Study the drawing (mm; zero at the part's minimum x, y, z) and answer. Round coordinates to 2 decimals unless told otherwise and drop trailing zeros. Loops run counter-clockwise (first coordinate to the right, second up) from the corner with the lowest first, then second, coordinate; pieces in that order, holes last. Notation, with made-up numbers: (85, -1.75) -> (102, -1.75) arc R27 cw to (102, 20.25) -> close; hole circle Ø1 at (84.25, 6.25). An arc over 180 degrees is marked (long way). Answer in a Markdown table with one row per item. Add a question column.
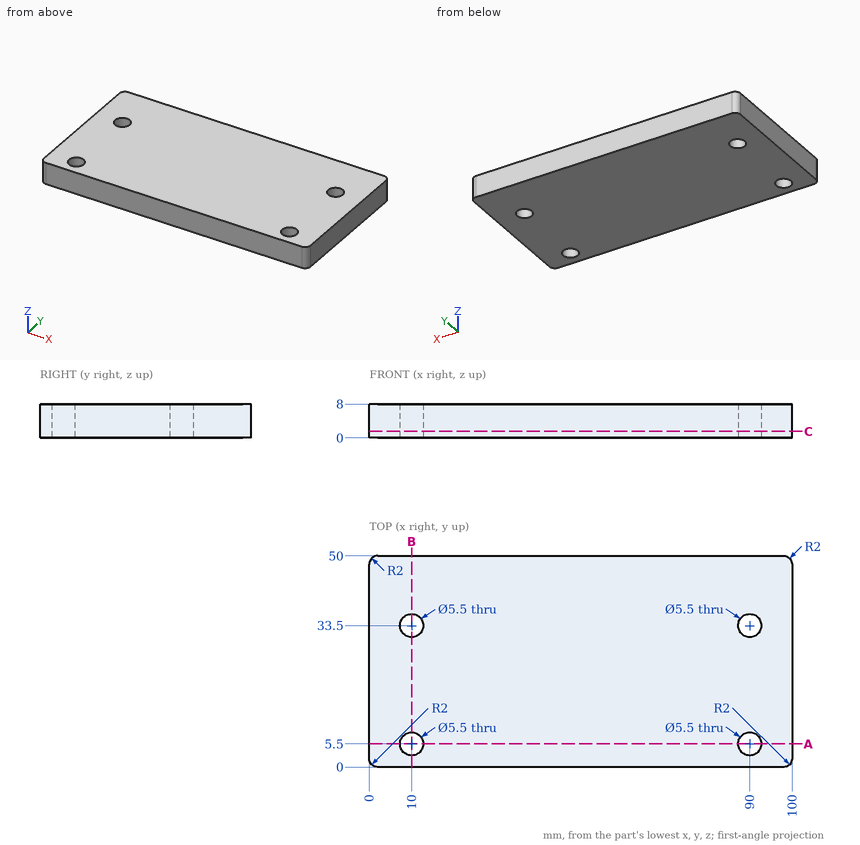
Item 1: Section A-A, the plane y = 5.5 is taken. Write down the section's boundary in (x, z).
Item 2: A flat-ended cylindrical pin translates along its axis: P1, Ø5, axis at x = 10, y = 33.5, coming from the -Z side. Find the tip coordinate at first contact, or state that the pin passes through.
Item 3: Section B-B, the plane x = 10 is taken. Write down the section's boundary in (y, z), and give its area (3 significant figures).
Item 4: Section C-C, the plane z = 1.5 is taken. Write down the section's boundary in (x, y), and give its area (3 significant figures).
Item 5: Consider L1, parallel to X at y = 33.5, z = 5; L2, parallel to Y at x = 90, z = 6; L3, parallel to X at y = 3, z = 0.5. Determine where each line is inside the solid, lowest interval first. Write a range as from..to.
Here are the results:
| question | item | result |
|---|---|---|
| 1 | outline | (0, 0) -> (7.25, 0) -> (7.25, 8) -> (0, 8) -> close; (12.75, 0) -> (87.25, 0) -> (87.25, 8) -> (12.75, 8) -> close; (92.75, 0) -> (100, 0) -> (100, 8) -> (92.75, 8) -> close |
| 2 | P1 | passes through |
| 3 | outline | (0, 0) -> (2.75, 0) -> (2.75, 8) -> (0, 8) -> close; (8.25, 0) -> (30.75, 0) -> (30.75, 8) -> (8.25, 8) -> close; (36.25, 0) -> (50, 0) -> (50, 8) -> (36.25, 8) -> close |
| 3 | area | 312 mm² |
| 4 | outline | (0, 2) arc R2 ccw to (2, 0) -> (98, 0) arc R2 ccw to (100, 2) -> (100, 48) arc R2 ccw to (98, 50) -> (2, 50) arc R2 ccw to (0, 48) -> close; hole circle Ø5.5 at (10, 5.5); hole circle Ø5.5 at (10, 33.5); hole circle Ø5.5 at (90, 5.5); hole circle Ø5.5 at (90, 33.5) |
| 4 | area | 4,900 mm² |
| 5 | L1 | x = 0..7.25, 12.75..87.25, 92.75..100 |
| 5 | L2 | y = 0..2.75, 8.25..30.75, 36.25..50 |
| 5 | L3 | x = 0..8.85, 11.15..88.85, 91.15..100 |
